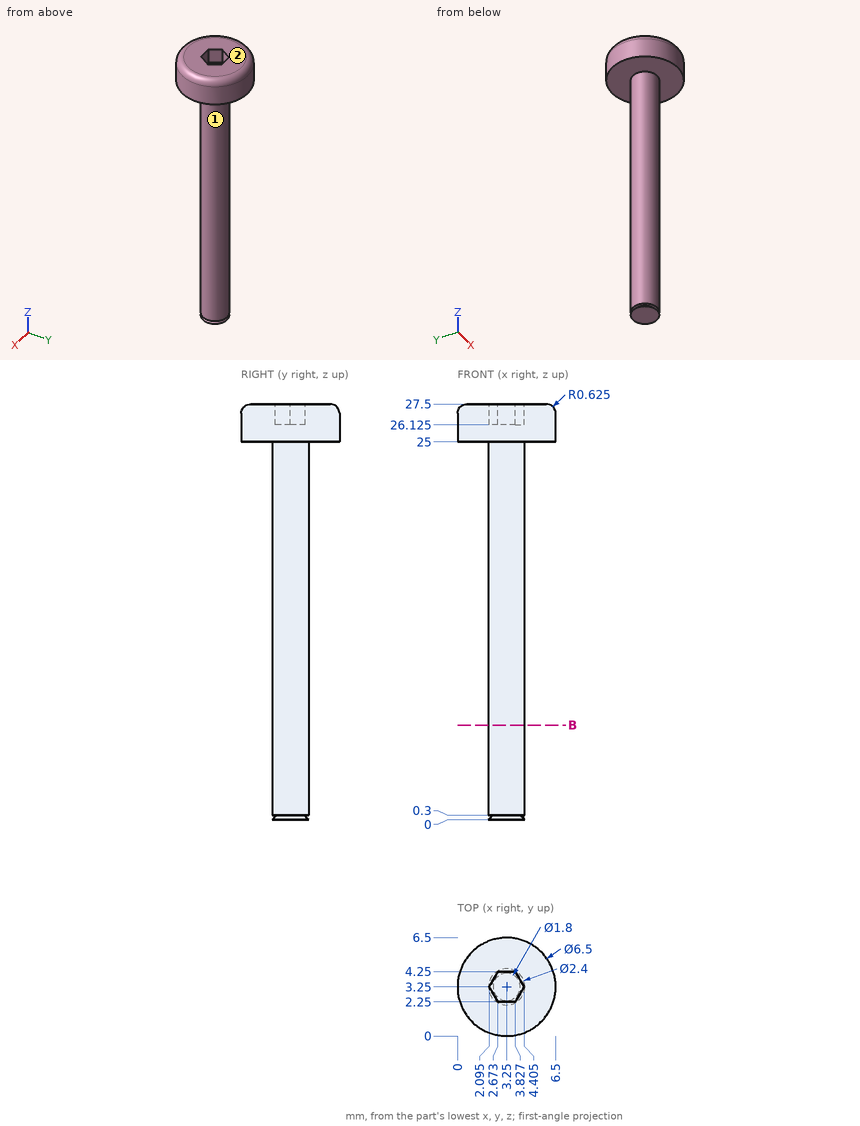
Could you check a few things on this drawing? It's one solid part, dimensions in mm from its lowest x, y, z. A direction names the side the tool comes from. Round coordinates to 2 decimals unless told otherwise and drop trailing zeros. Write each loop counter-clockwise with the first axis right and the second up, starting at its lowest first coordinate (ties: lowest second). Pieces come first, ordered by that corner, then holes. Notation, with made-up numbers: M 14.5,75.5 L 33.5,75.5 A17 ccw 33.5,84.5 Z; hole C -37,23 d9. An arc over 180 degrees is marked long. Answer as CSV lines item,"result". Start each with the question number.
1. On a 3-axis mill with a long thin cutter (end or side, diameter ignored), from which of +Z, -Z, +X, -X, +Y, -Y can I reach the whole of each face in a straight line? I mean the marked faces 1 and 2. Say none if no direction works.
2. Suppose I cut it at B-B on z = 6.25. Write out the boundary of the cut face in (x, y).
3. I'm going to push a flat-ended pin straight in: pin 1 Ø2 at (y, z) = (3, 20.5) entering from -X. Where does the tip first touch, or does it pass through?
4. I need wall thicknesses on probe 1 along Y at (x, z) = (3, 26.25); probe 2 along Z at (x, y) = (2, 2.25); probe 3 along X at (y, z) = (3.5, 8). Which ranges of each line are inside material? Lowest first, please.
Check result:
1,face 1,"-Z"
1,face 2,"+Z, +X, -X, +Y, -Y"
2,outline,"C 3.25,3.25 d2.4"
3,pin 1,"stops at x = 2.05"
4,probe 1,"y = 0.01 to 2.25, 4.25 to 6.49"
4,probe 2,"z = 25 to 27.5"
4,probe 3,"x = 2.08 to 4.42"
